Design review of the part built by this model. Coordinates are the model's own, in mm. Face numbers are marked on the shaded views. Round coordinates to 2 decimals unless told otherwise and drop trailing zeros. Loops run counter-clockwise (first coordinate to the right, second up) from the corner with the lowest first, then second, coordinate; pieces in that order, holes last. Notation, with made-up numbers: (5, -35.5) -> (38, -35.5) arc R19 ccw to (38, -31.5) -> close; hole circle Ø8 at (72, 10.5). An arc over 180 degrees is marked (long way). Answer as CSV lines item,"result". Start each with the question number.
(1) Draft analysis for pull direction X (two halves, no side actions). For the marked faces 1, 2 and 3, state which applies: +X half, -X half, draft (parallel to the pull), parting line (faces both ways), or undercut.
(2) Take a section at C-C, the plane z = 11.5. State how many separate pieces and enclosed holes the cut face has, and give its area (3 significant figures).
(3) Take a section at A-A, the plane x = 0. Write out the cut boundary in (y, z).
(4) For P1, Ø1, axis at y = -18.5, z = 18.5, coming from the +X side; P2, Ø10, axis at y = -27, z = -4, coming from the -X side; P3, Ø4, axis at x = 25.5, z = 17, coming from the +Y side, all flat-tipped, find the tip position at first contact; note any pin that passes through.
(5) To check wall thickness, follow line 1 (Y direction, x = -58, z = -6) (3 decimals); line 2 (Y direction, x = 42.5, z = -8); line 3 (X direction, y = 42, z = -2.5). State the ranges of each line that lie inside material, in increasing order. Write a range as from..to.
from build123d import *

# Parameters (mm, degrees)
ACTUATOR_HOUSING_MOUNT_R    = 64.3
ACTUATOR_HOUSING_MOUNT_R_2  = 55.8
ACTUATOR_HOUSING_MOUNT_R_3  = 1.55
ACTUATOR_HOUSING_WALL_DEPTH = 25
SKETCH2_R                   = 64.3
SKETCH2_R_2                 = 1.55
SKETCH2_R_3                 = 55.8
BOSS_EXTRUDE2_DEPTH         = 5
CUT_EXTRUDE1_START          = -5
SKETCH3_R                   = 11.55
CUT_EXTRUDE1_DEPTH          = 4
SKETCH4_R                   = 11
CUT_EXTRUDE2_DEPTH          = 4
BOSS_EXTRUDE3_START         = 8
SKETCH6_R                   = 64.3
SKETCH6_R_2                 = 63.25
BOSS_EXTRUDE3_DEPTH         = 8
SKETCH7_R                   = 2
M3_INSERT_L12_DEPTH         = 12
CHAMFER2_SIZE               = 0.5


with BuildPart() as part:
    # Actuator Housing Mount → Actuator Housing Wall (new body)
    with BuildSketch(Plane.XY.offset(19)):
        Circle(ACTUATOR_HOUSING_MOUNT_R)
        Circle(ACTUATOR_HOUSING_MOUNT_R_2, mode=Mode.SUBTRACT)
        with Locations((57.375994082, 15.373851279)):
            Circle(ACTUATOR_HOUSING_MOUNT_R_3, mode=Mode.SUBTRACT)
        with Locations((57.375994082, -15.373851279)):
            Circle(ACTUATOR_HOUSING_MOUNT_R_3, mode=Mode.SUBTRACT)
        with Locations((42.002142802, -42.002142802)):
            Circle(ACTUATOR_HOUSING_MOUNT_R_3, mode=Mode.SUBTRACT)
        with Locations((15.373851279, -57.375994082)):
            Circle(ACTUATOR_HOUSING_MOUNT_R_3, mode=Mode.SUBTRACT)
        with Locations((-15.373851279, -57.375994082)):
            Circle(ACTUATOR_HOUSING_MOUNT_R_3, mode=Mode.SUBTRACT)
        with Locations((-42.002142802, -42.002142802)):
            Circle(ACTUATOR_HOUSING_MOUNT_R_3, mode=Mode.SUBTRACT)
        with Locations((-57.375994082, -15.373851279)):
            Circle(ACTUATOR_HOUSING_MOUNT_R_3, mode=Mode.SUBTRACT)
        with Locations((-57.375994082, 15.373851279)):
            Circle(ACTUATOR_HOUSING_MOUNT_R_3, mode=Mode.SUBTRACT)
        with Locations((-42.002142802, 42.002142802)):
            Circle(ACTUATOR_HOUSING_MOUNT_R_3, mode=Mode.SUBTRACT)
        with Locations((-15.373851279, 57.375994082)):
            Circle(ACTUATOR_HOUSING_MOUNT_R_3, mode=Mode.SUBTRACT)
        with Locations((15.373851279, 57.375994082)):
            Circle(ACTUATOR_HOUSING_MOUNT_R_3, mode=Mode.SUBTRACT)
        with Locations((42.002142802, 42.002142802)):
            Circle(ACTUATOR_HOUSING_MOUNT_R_3, mode=Mode.SUBTRACT)
    extrude(amount=-ACTUATOR_HOUSING_WALL_DEPTH)

    # Sketch2 → Boss-Extrude2 (add)
    # profile 1 of 2: a face of its own
    with BuildSketch(Plane(origin=(0, 0, -6), x_dir=(-1, 0, 0), z_dir=(0, 0, -1))):
        with Locations(Location((0, 0, 0), (0, 0, 180))):
            Circle(SKETCH2_R)
        with Locations(Location((-15.373851279, 57.375994082, 0), (0, 0, 180))):
            Circle(SKETCH2_R_2, mode=Mode.SUBTRACT)
        with Locations(Location((42.002142802, 42.002142802, 0), (0, 0, 180))):
            Circle(SKETCH2_R_2, mode=Mode.SUBTRACT)
        with Locations(Location((57.375994082, -15.373851279, 0), (0, 0, 180))):
            Circle(SKETCH2_R_2, mode=Mode.SUBTRACT)
        with Locations(Location((15.373851279, -57.375994082, 0), (0, 0, 180))):
            Circle(SKETCH2_R_2, mode=Mode.SUBTRACT)
        with Locations(Location((-42.002142802, -42.002142802, 0), (0, 0, 180))):
            Circle(SKETCH2_R_2, mode=Mode.SUBTRACT)
        with Locations(Location((-57.375994082, -15.373851279, 0), (0, 0, 180))):
            Circle(SKETCH2_R_2, mode=Mode.SUBTRACT)
        with Locations(Location((-57.375994082, 15.373851279, 0), (0, 0, 180))):
            Circle(SKETCH2_R_2, mode=Mode.SUBTRACT)
        with Locations(Location((0, 0, 0), (0, 0, 180))):
            Circle(SKETCH2_R_3, mode=Mode.SUBTRACT)
        with Locations(Location((-15.373851279, -57.375994082, 0), (0, 0, 180))):
            Circle(SKETCH2_R_2, mode=Mode.SUBTRACT)
        with Locations(Location((42.002142802, -42.002142802, 0), (0, 0, 180))):
            Circle(SKETCH2_R_2, mode=Mode.SUBTRACT)
        with Locations(Location((57.375994082, 15.373851279, 0), (0, 0, 180))):
            Circle(SKETCH2_R_2, mode=Mode.SUBTRACT)
        with Locations(Location((15.373851279, 57.375994082, 0), (0, 0, 180))):
            Circle(SKETCH2_R_2, mode=Mode.SUBTRACT)
        with Locations(Location((-42.002142802, 42.002142802, 0), (0, 0, 180))):
            Circle(SKETCH2_R_2, mode=Mode.SUBTRACT)
    # profile 2 of 2: a face of its own
    with BuildSketch(Plane(origin=(0, 0, -6), x_dir=(-1, 0, 0), z_dir=(0, 0, -1))):
        with Locations(Location((0, 0, 0), (0, 0, 180))):
            Circle(SKETCH2_R_3)
    extrude(amount=BOSS_EXTRUDE2_DEPTH)

    # Sketch3 → Cut-Extrude1 (cut)
    with BuildSketch(Plane(origin=(0, 0, -11), x_dir=(-1, 0, 0), z_dir=(0, 0, -1)).offset(CUT_EXTRUDE1_START)):
        Circle(SKETCH3_R)
    extrude(amount=CUT_EXTRUDE1_DEPTH, mode=Mode.SUBTRACT)

    # Sketch4 → Cut-Extrude2 (cut)
    with BuildSketch(Plane(origin=(0, 0, -11), x_dir=(-1, 0, 0), z_dir=(0, 0, -1))):
        Circle(SKETCH4_R)
    extrude(amount=-CUT_EXTRUDE2_DEPTH, mode=Mode.SUBTRACT)

    # Sketch6 → Boss-Extrude3 (add)
    with BuildSketch(Plane.XY.offset(19).offset(BOSS_EXTRUDE3_START)):
        Circle(SKETCH6_R)
        Circle(SKETCH6_R_2, mode=Mode.SUBTRACT)
    extrude(amount=-BOSS_EXTRUDE3_DEPTH)

    # Sketch7 → M3 Insert L12 (cut)
    with BuildSketch(Plane.XY.offset(19)):
        with Locations((57.375994082, -15.373851279)):
            Circle(SKETCH7_R)
        with Locations((42.002142802, -42.002142802)):
            Circle(SKETCH7_R)
        with Locations((15.373851279, -57.375994082)):
            Circle(SKETCH7_R)
        with Locations((-15.373851279, -57.375994082)):
            Circle(SKETCH7_R)
        with Locations((-42.002142802, -42.002142802)):
            Circle(SKETCH7_R)
        with Locations((-57.375994082, -15.373851279)):
            Circle(SKETCH7_R)
        with Locations((-57.375994082, 15.373851279)):
            Circle(SKETCH7_R)
        with Locations((-42.002142802, 42.002142802)):
            Circle(SKETCH7_R)
        with Locations((-15.373851279, 57.375994082)):
            Circle(SKETCH7_R)
        with Locations((15.373851279, 57.375994082)):
            Circle(SKETCH7_R)
        with Locations((42.002142802, 42.002142802)):
            Circle(SKETCH7_R)
        with Locations((57.375994082, 15.373851279)):
            Circle(SKETCH7_R)
    extrude(amount=-M3_INSERT_L12_DEPTH, mode=Mode.SUBTRACT)

    # Chamfer2
    chamfer2_edges = [part.edges().sort_by_distance(p)[0] for p in [
        (-64.3, 0, 27),
        (-64.3, 0, -11),
    ]]
    chamfer(chamfer2_edges, length=CHAMFER2_SIZE)


solid = part.part
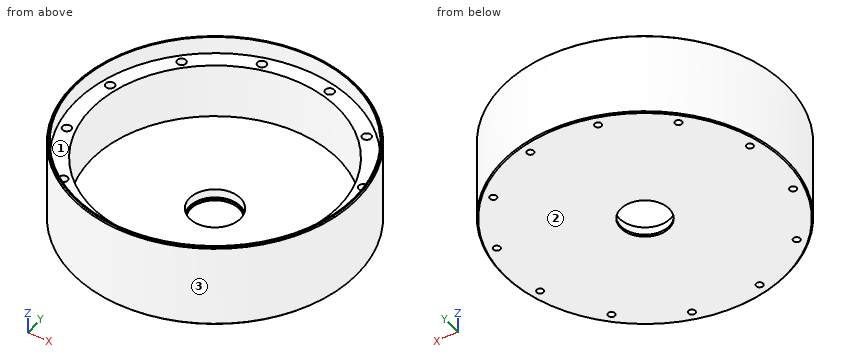
The answers:
1,face 1,"undercut"
1,face 2,"draft"
1,face 3,"parting line"
2,separate pieces,"1"
2,enclosed holes,"13"
2,area,"3,060 mm²"
3,outline,"(-64.3, -10.5) -> (-63.8, -11) -> (-11, -11) -> (-11, -10) -> (-11.55, -10) -> (-11.55, -6) -> (-55.8, -6) -> (-55.8, 19) -> (-63.25, 19) -> (-63.25, 27) -> (-63.8, 27) -> (-64.3, 26.5) -> close; (11, -11) -> (63.8, -11) -> (64.3, -10.5) -> (64.3, 26.5) -> (63.8, 27) -> (63.25, 27) -> (63.25, 19) -> (55.8, 19) -> (55.8, -6) -> (11.55, -6) -> (11.55, -10) -> (11, -10) -> close"
4,P1,"x = 61.73"
4,P2,"x = -60.42"
4,P3,"y = 59.85"
5,line 1,"-27.758..-16.793, -13.955..13.955, 16.793..27.758"
5,line 2,"-48.25..-43.47, -40.53..40.53, 43.47..48.25"
5,line 3,"-48.69..-43.55, -40.45..-36.74, 36.74..40.45, 43.55..48.69"
